```python
from build123d import *

# Parameters (mm, degrees)
SKETCH1_W            = 261.9
SKETCH1_H            = 61.9
SKETCH1_H_2          = 161.9
BOSS_EXTRUDE1_DEPTH  = 38.1
SHELL1_START         = 3.175
SHELL1_OUTLINE_W     = 31.75
SHELL1_OUTLINE_H     = 31.75
SHELL1_DEPTH         = 2162.7
SHELL1_START_2       = 1834.125
SHELL1_2_OUTLINE_W   = 31.75
SHELL1_2_OUTLINE_H   = 31.75
SHELL1_2_DEPTH       = 331.75
SHELL1_START_3       = 484.125
SHELL1_3_OUTLINE_W   = 600
SHELL1_3_OUTLINE_H   = 31.75
SHELL1_3_DEPTH       = 31.75
SHELL1_4_OUTLINE_W   = 68.25
SHELL1_4_OUTLINE_H   = 31.75
SHELL1_4_OUTLINE_W_2 = 168.25
SHELL1_4_DEPTH       = 31.75
SHELL1_START_4       = 2134.125
SHELL1_5_OUTLINE_W   = 68.25
SHELL1_5_OUTLINE_H   = 31.75
SHELL1_5_OUTLINE_W_2 = 168.25
SHELL1_5_DEPTH       = 31.75


# Read off the part's stored shape, not the designer's step: Shell1
with BuildPart() as part:
    # Sketch1 → Boss-Extrude1 (new body)
    with BuildSketch(Plane.XY):
        Polygon((0, 0), (2169.05, 0), (2169.05, 38.1), (2169.05, 138.1), (2169.05, 338.1), (1869.05, 338.1), (1830.95, 338.1), (1830.95, 38.1), (519.05, 38.1), (519.05, 638.1), (480.95, 638.1), (480.95, 38.1), (0, 38.1), align=None)
        with Locations((2000, 69.05)):
            Rectangle(SKETCH1_W, SKETCH1_H, mode=Mode.SUBTRACT)
        with Locations((2000, 219.05)):
            Rectangle(SKETCH1_W, SKETCH1_H_2, mode=Mode.SUBTRACT)
    extrude(amount=-BOSS_EXTRUDE1_DEPTH)

    # Shell1 outline → Shell1 (cut)
    with BuildSketch(Plane.YZ.offset(SHELL1_START)):
        with Locations((19.05, -19.05)):
            Rectangle(SHELL1_OUTLINE_W, SHELL1_OUTLINE_H)
    extrude(amount=SHELL1_DEPTH, mode=Mode.SUBTRACT)

    # Shell1 2 outline → Shell1 2 (cut)
    with BuildSketch(Plane.YZ.offset(SHELL1_START_2)):
        with Locations((119.05, -19.05)):
            Rectangle(SHELL1_2_OUTLINE_W, SHELL1_2_OUTLINE_H)
        with Locations((319.05, -19.05)):
            Rectangle(SHELL1_2_OUTLINE_W, SHELL1_2_OUTLINE_H)
    extrude(amount=SHELL1_2_DEPTH, mode=Mode.SUBTRACT)

    # Shell1 3 outline → Shell1 3 (cut)
    with BuildSketch(Plane.YZ.offset(SHELL1_START_3)):
        with Locations((334.925, -19.05)):
            Rectangle(SHELL1_3_OUTLINE_W, SHELL1_3_OUTLINE_H)
    extrude(amount=SHELL1_3_DEPTH, mode=Mode.SUBTRACT)

    # Shell1 4 outline → Shell1 4 (cut)
    with BuildSketch(Plane.YZ.offset(SHELL1_START_2)):
        with Locations((69.05, -19.05)):
            Rectangle(SHELL1_4_OUTLINE_W, SHELL1_4_OUTLINE_H)
        with Locations((219.05, -19.05)):
            Rectangle(SHELL1_4_OUTLINE_W_2, SHELL1_4_OUTLINE_H)
    extrude(amount=SHELL1_4_DEPTH, mode=Mode.SUBTRACT)

    # Shell1 5 outline → Shell1 5 (cut)
    with BuildSketch(Plane.YZ.offset(SHELL1_START_4)):
        with Locations((69.05, -19.05)):
            Rectangle(SHELL1_5_OUTLINE_W, SHELL1_5_OUTLINE_H)
        with Locations((219.05, -19.05)):
            Rectangle(SHELL1_5_OUTLINE_W_2, SHELL1_5_OUTLINE_H)
    extrude(amount=SHELL1_5_DEPTH, mode=Mode.SUBTRACT)


solid = part.part
```
Geometry check sheet. Reference: the model listing, model coordinates, mm. A direction names the side the tool comes from. Round coordinates to 2 decimals unless told otherwise and drop trailing zeros. Order: outer loops, then holes, each group sorted by start corner. A loop starts at its lowest first (then second) coordinate and runs counter-clockwise, first axis right, second up. Notation, with made-up numbers: (45.5, -9.75) -> (64.5, -9.75) arc R22 cw to (64.5, 23.25) -> close; hole circle Ø5 at (-1.75, -22). An arc over 180 degrees is marked (long way). Return JSON: item names as keys, results as strings. Group by question number.
Q1. Gauge pin test, flat ends, axial feed: pin 1 (19 mm diameter, centred on x = 1929.5, z = -17, fed in from +Y); pin 2 (10 mm diameter, centred on y = 352, z = -14.5, fed in from -X). Record the tip position at first contact, or that the pin passes through.
Q2. Section check D-D, the plane y = 439. Record the boundary of the cut face in (x, z) (3 decimals).
Q3. Section check C-C, the plane z = -14. Count the separate pieces of the cut face and the enclosed holes in it, plus the area to 3 significant figures.
Q4. Section check B-B, the plane x = 793. Record the boundary of the cut face in (y, z) (3 decimals).
Q5. Material ranges on probe 1 along X at (y, z) = (62.5, -23) (3 decimals); probe 2 along Y at (x, z) = (1905.5, -31) (3 decimals); probe 3 along X at (y, z) = (106, -22) (3 decimals), recorded low to high. Write a range as from..to.
Q6. Section check A-A, the plane y = 261.5. Record the boundary of the cut face in (x, z) (3 decimals), plus the area to 3 significant figures.
Q7. Tool access check on faces 1 (the flat face through (480.95, 342, -19)), 2 (the flat face through (519.05, 334, -19)), 3 (the flat face through (1998, 38.1, -19)). Record the directions out of +Z, -Z, +X, -X, +Y, -Y that give a thin tool (end or side, any length) a straight path to the whole face; none if there is none.
Q8. Release check for a two-part mould opening along Y. For faces 4 (the flat face through (1830.95, 190, -19)), 5 (the flat face through (1069, 0, -19)), 6 (the flat face through (1998, 138.1, -19)) record: released by +Y, released by -Y, zero draft, split by the parting line, or undercut.
Numbers:
{
 "1": {"pin 1": "y = 338.1", "pin 2": "x = 480.95"},
 "2": {"outline": "(480.95, -38.1) -> (519.05, -38.1) -> (519.05, 0) -> (480.95, 0) -> close; hole (484.125, -34.925) -> (515.875, -34.925) -> (515.875, -3.175) -> (484.125, -3.175) -> close"},
 "3": {"separate pieces": "3", "enclosed holes": "3", "area": "24,500 mm^2"},
 "4": {"outline": "(0, -38.1) -> (38.1, -38.1) -> (38.1, 0) -> (0, 0) -> close; hole (3.175, -34.925) -> (34.925, -34.925) -> (34.925, -3.175) -> (3.175, -3.175) -> close"},
 "5": {"probe 1": "480.95..484.125, 515.875..519.05, 1830.95..1834.125, 1865.875..1869.05, 2130.95..2134.125, 2165.875..2169.05", "probe 2": "0..3.175, 34.925..38.1, 100..103.175, 134.925..138.1, 300..303.175, 334.925..338.1", "probe 3": "480.95..484.125, 515.875..519.05, 1830.95..1834.125, 2165.875..2169.05"},
 "6": {"outline": "(480.95, -38.1) -> (519.05, -38.1) -> (519.05, 0) -> (480.95, 0) -> close; (1830.95, -38.1) -> (1869.05, -38.1) -> (1869.05, 0) -> (1830.95, 0) -> close; (2130.95, -38.1) -> (2169.05, -38.1) -> (2169.05, 0) -> (2130.95, 0) -> close; hole (484.125, -34.925) -> (515.875, -34.925) -> (515.875, -3.175) -> (484.125, -3.175) -> close; hole (1834.125, -34.925) -> (1865.875, -34.925) -> (1865.875, -3.175) -> (1834.125, -3.175) -> close; hole (2134.125, -34.925) -> (2165.875, -34.925) -> (2165.875, -3.175) -> (2134.125, -3.175) -> close", "area": "1,330 mm^2"},
 "7": {"face 1": "+Z, -Z, -X, +Y", "face 2": "+Z, -Z, +Y", "face 3": "+Z, -Z"},
 "8": {"face 4": "zero draft", "face 5": "released by -Y", "face 6": "undercut"}
}
